Geometry: see drawing. Coordinates: mm, zero at the bounding-box minimum. A direction names the side the tool comes from. Coordinates: 2 decimals unless noted, no trailing zeros. Loops run counter-clockwise (first coordinate to the right, second up) from the corner with the lowest first, then second, coordinate; pieces in that order, holes last. Notation, with made-up numbers: M 22,-33.5 L 52,-33.5 A23 cw 52,-5.5 Z; hole C -35.5,-4 d7. An arc over 180 degrees is marked long. One line per question, with ' | ' between items. Start each with the question number.
1. Pin query (flat end, axial travel): P1, Ø4, axis at x = 33, z = 34, coming from the -Y side. Return the tip coordinate at first contact, or that it passes through.
2. Access query for the marked faces 1 and 2. Directions: +Z, -Z, +X, -X, +Y, -Y. A direction counts if a zero-diameter tool reaches every point of the face in a straight line with its end or side. Return the directions, or none.
3. Ray query, probe 1 along X at (y, z) = (9.5, 19.05) (3 decimals); probe 2 along Z at (x, y) = (44.45, 10); probe 3 along X at (y, z) = (6.25, 25.5). Return the intervals inside material, ascending.
4. Mould query, pull axis X, two halves, no side actions, for the marked faces 3, 4 and 5. Classes: pulls with the +X half, pulls with the -X half, needs draft (parallel to the pull), parting line crosses it, or undercut.
5. Section query D-D, the plane z = 35. Output: boundary loops of the cut face in (x, y) (3 decimals).
6. Section query B-B, the plane x = 19.05. Output: boundary loops of the cut face in (y, z).
7. Section query A-A, the plane y = 3.5. Output: boundary loops of the cut face in (x, z), and give its area (3 significant figures).
8. Section query C-C, the plane z = 19.05. Output: boundary loops of the cut face in (x, y) (3 decimals), and give its area (3 significant figures).
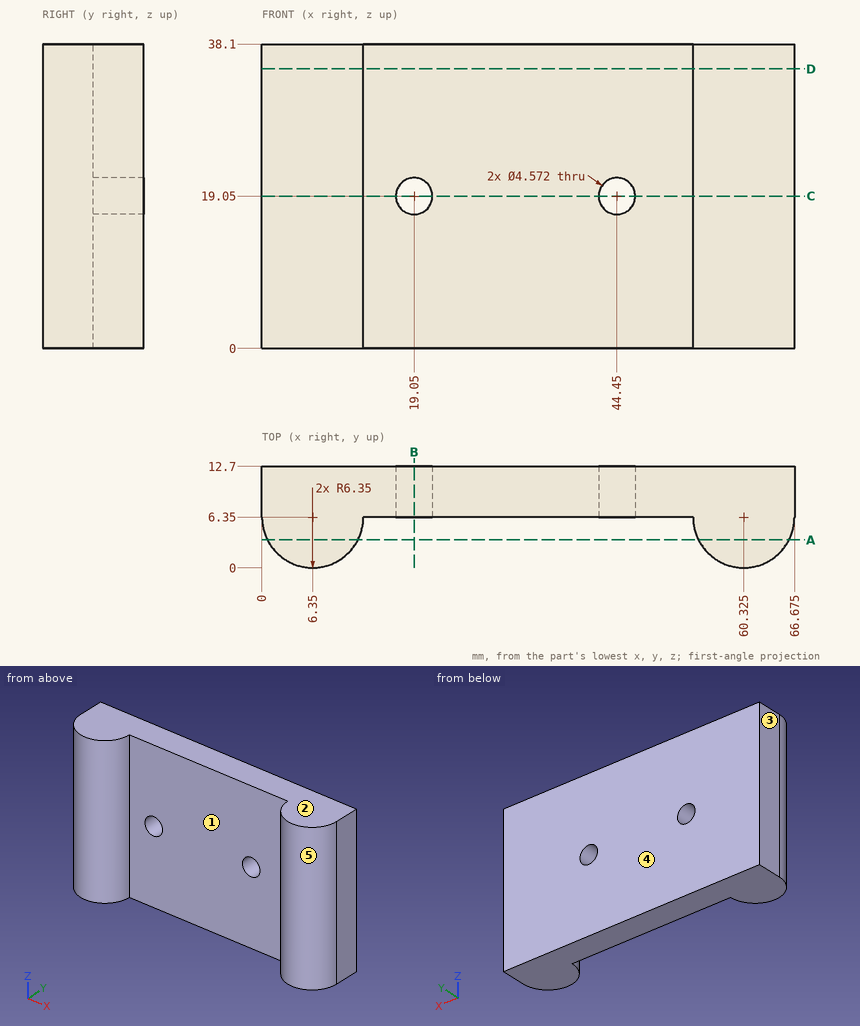
Taken from the geometry:
1) P1: y = 6.35
2) face 1: +Z, -Z, -Y | face 2: +Z, +X, -X, +Y, -Y
3) probe 1: 0 to 16.764, 21.336 to 42.164, 46.736 to 66.675 | probe 2: 0 to 16.76, 21.34 to 38.1 | probe 3: 0 to 12.7, 53.98 to 66.67
4) face 3: pulls with the -X half | face 4: needs draft | face 5: undercut
5) outline: M 0,6.35 A6.35 ccw 12.7,6.35 L 53.975,6.35 A6.35 ccw 66.675,6.35 L 66.675,12.7 L 0,12.7 Z
6) outline: M 6.35,0 L 12.7,0 L 12.7,16.76 L 6.35,16.76 Z; M 6.35,21.34 L 12.7,21.34 L 12.7,38.1 L 6.35,38.1 Z
7) outline: M 0.68,0 L 12.02,0 L 12.02,38.1 L 0.68,38.1 Z; M 54.65,0 L 66,0 L 66,38.1 L 54.65,38.1 Z | area: 865 mm^2
8) outline: M 0,6.35 A6.35 ccw 12.7,6.35 L 16.764,6.35 L 16.764,12.7 L 0,12.7 Z; M 21.336,6.35 L 42.164,6.35 L 42.164,12.7 L 21.336,12.7 Z; M 46.736,6.35 L 53.975,6.35 A6.35 ccw 66.675,6.35 L 66.675,12.7 L 46.736,12.7 Z | area: 492 mm^2
